from build123d import *

# Parameters (mm, degrees)
CROQUIS1_W               = 100
CROQUIS1_H               = 15
SALIENTE_EXTRUIR1_DEPTH  = 50
CROQUIS17_R              = 30
CORTAR_EXTRUIR1_DEPTH    = 15
BARRER1_PROFILE_R        = 35
CORTAR_BARRER2_PROFILE_R = 30
REDONDEO1_R              = 15
TALADRO1_D               = 15
TALADRO1_DEPTH           = 15
CROQUIS26_W              = 100
CROQUIS26_H              = 100
SALIENTE_EXTRUIR3_DEPTH  = 15
REDONDEO2_R              = 15
CROQUIS29_R              = 30
CORTAR_EXTRUIR2_DEPTH    = 15
TALADRO2_D               = 15
TALADRO2_DEPTH           = 15
TALADRO2_ON_FACE_2_D     = 15
TALADRO2_ON_FACE_2_DEPTH = 15


with BuildPart() as part:
    # Croquis1 → Saliente-Extruir1 (new, symmetric)
    with BuildSketch(Plane.XY):
        with Locations((0, 7.5)):
            Rectangle(CROQUIS1_W, CROQUIS1_H)
    extrude(amount=SALIENTE_EXTRUIR1_DEPTH, both=True)

    # Croquis17 → Cortar-Extruir1 (cut)
    with BuildSketch(Plane(origin=(0, 15, 0), x_dir=(1, 0, 0), z_dir=(0, 1, 0))):
        with Locations(Location((0, 0, 0), (0, 0, 180))):
            Circle(CROQUIS17_R)
    extrude(amount=-CORTAR_EXTRUIR1_DEPTH, mode=Mode.SUBTRACT)

    # Barrer1: sweep along a path in Croquis2
    with BuildLine(Plane.XY) as barrer1_path:
        Line((0, 0), (0, 61.152236891))
        ThreePointArc((0, 61.152236891), (9.895660774, 110.901083099), (38.076118446, 153.076118446))
        Line((38.076118446, 153.076118446), (70.710678119, 185.710678119))
    # Barrer1 profile (on start of the path) → Barrer1 (sweep)
    with BuildSketch(Plane(origin=(0, 0, 0), x_dir=(1, 0, 0), z_dir=(0, 1, 0))):
        Circle(BARRER1_PROFILE_R)
    sweep(path=barrer1_path.line)

    # Cortar-Barrer2: sweep along a path in Croquis2<5>
    with BuildLine(Plane.XY) as cortar_barrer2_path:
        Line((0, 0), (0, 61.152236891))
        ThreePointArc((0, 61.152236891), (9.895660774, 110.901083099), (38.076118446, 153.076118446))
        Line((38.076118446, 153.076118446), (70.710678119, 185.710678119))
    # Cortar-Barrer2 profile (on start of the path) → Cortar-Barrer2 (sweep, cut)
    with BuildSketch(Plane(origin=(0, 0, 0), x_dir=(1, 0, 0), z_dir=(0, 1, 0))):
        Circle(CORTAR_BARRER2_PROFILE_R)
    sweep(path=cortar_barrer2_path.line, mode=Mode.SUBTRACT)

    # Redondeo1
    redondeo1_edges = [part.edges().sort_by_distance(p)[0] for p in [
        (50, 7.5, 50),
        (-50, 7.5, 50),
        (50, 7.5, -50),
        (-50, 7.5, -50),
    ]]
    fillet(redondeo1_edges, radius=REDONDEO1_R)

    # Taladro1
    with Locations(Plane(origin=(-35, 15, -35), x_dir=(1, 0, 0), z_dir=(0, 1, 0))):
        with Locations((0, 0), (0, -70), (70, 0), (70, -70)):
            Hole(TALADRO1_D / 2, depth=TALADRO1_DEPTH)

    # Croquis26 → Saliente-Extruir3 (add)
    with BuildSketch(Plane(origin=(128.210678119, 128.210678119, 0), x_dir=(0, 0, -1), z_dir=(0.7071067811865478, 0.7071067811865472, 0))):
        with Locations((0, 81.317279836)):
            Rectangle(CROQUIS26_W, CROQUIS26_H)
    extrude(amount=SALIENTE_EXTRUIR3_DEPTH)

    # Redondeo2
    redondeo2_edges = [part.edges().sort_by_distance(p)[0] for p in [
        (40.658639918, 226.369318037, 50),
        (111.369318037, 155.658639918, 50),
        (111.369318037, 155.658639918, -50),
        (40.658639918, 226.369318037, -50),
    ]]
    fillet(redondeo2_edges, radius=REDONDEO2_R)

    # Croquis29 → Cortar-Extruir2 (cut)
    with BuildSketch(Plane(origin=(138.817279836, 138.817279836, 0), x_dir=(0, 0, -1), z_dir=(0.7071067811865479, 0.7071067811865472, 0))):
        with Locations(Location((0, 81.317279836, 0), (0, 0, 90))):
            Circle(CROQUIS29_R)
    extrude(amount=-CORTAR_EXTRUIR2_DEPTH, mode=Mode.SUBTRACT)

    # Taladro2
    with Locations(Plane(origin=(56.568542495, 221.066017178, 35), x_dir=(-0.707106781187, 0.707106781187, 0), z_dir=(0.707106781187, 0.707106781187, 0))):
        with Locations((0, 0)):
            Hole(TALADRO2_D / 2, depth=TALADRO2_DEPTH)

    # Taladro2 on face 2
    with Locations(Plane(origin=(106.066017178, 171.568542495, 35), x_dir=(0.707106781187, -0.707106781187, 0), z_dir=(0.707106781187, 0.707106781187, 0))):
        with Locations((0, 0), (0, 70), (-70, 70)):
            Hole(TALADRO2_ON_FACE_2_D / 2, depth=TALADRO2_ON_FACE_2_DEPTH)


solid = part.part
Build history of the part. All positions in model axes, mm. A direction names the side the tool comes from. Give positions to 0.01 mm unless a question says otherwise; leave off trailing zeros. Loops run counter-clockwise (first coordinate to the right, second up) from the corner with the lowest first, then second, coordinate; pieces in that order, holes last. Notation, with made-up numbers: (62, 34) -> (80, 34) arc R27 ccw to (80, 55) -> close; hole circle Ø11 at (-28.5, 29.5). An arc over 180 degrees is marked (long way). Answer in a Markdown table with one row per item.
Item 1: Slice it at B-B on y = 45. Write the cut outline in (x, z), plus the area to 3 significant figures.
Findings below:
| item | result |
|---|---|
| outline | circle Ø70 at (0, 0); hole circle Ø60 at (0, 0) |
| area | 1,020 mm² |
Item 2: Probe line 1 along Z through (x, y) = (-35, 4); line 2 along Y through (x, z) = (44, -2.5). List the from-to ranges inside material, lowest first. Write a range as [from, to].
Findings below:
| item | result |
|---|---|
| line 1 | z = [-50, -42.5], [-27.5, 27.5], [42.5, 50] |
| line 2 | y = [0, 15], [101.72, 112.39], [201.28, 208.37], [212.42, 229.71] |
Item 3: Mould opens along Z. For faces 5 (the cylindrical face through (36.63, 7.4, -27.68)), 6 (the cylindrical face through (108.42, 158.76, -45.49)), 7 (the cylindrical face through (108.254, 158.922, 45.723)) say: pulls with the +Z half, pulls with the -Z half, needs draft (parallel to the pull), parting line crosses it, or undercut.
Findings below:
| item | result |
|---|---|
| face 5 | undercut |
| face 6 | pulls with the -Z half |
| face 7 | pulls with the +Z half |
Item 4: Flat gauge pins, fed straight in: P1, Ø1.5, axis at y = 64.5, z = 24, coming from the -X side; P2, Ø1, axis at y = 141.5, z = -25.5, coming from the +X side; P3, Ø13.5, axis at x = -35, z = -35, coming from the +Y side; P4, Ø10, axis at x = -5, y = 118.5, coming from the +Z side. Where does each tip first touch, or does it go through?
Findings below:
| item | result |
|---|---|
| P1 | stops at x = -26.13 |
| P2 | stops at x = 61.3 |
| P3 | passes through |
| P4 | stops at z = 33 |
Item 5: Slice it at A-A on z = -8.5. Write the cut outline in (x, y), plus the area to 3 significant figures.
Findings below:
| item | result |
|---|---|
| outline | (-50, 0) -> (-28.77, 0) -> (-28.77, 61.15) arc R158.77 cw to (17.73, 173.42) -> (60.97, 216.66) -> (45.96, 231.67) -> (35.36, 221.07) -> (46.7, 209.72) -> (14.07, 177.08) arc R163.95 ccw to (-33.95, 61.15) -> (-33.95, 15) -> (-50, 15) -> close; (28.77, 0) -> (50, 0) -> (50, 15) -> (33.95, 15) -> (33.95, 61.15) arc R96.05 cw to (62.08, 129.07) -> (94.72, 161.7) -> (106.07, 150.36) -> (116.67, 160.96) -> (101.66, 175.97) -> (58.42, 132.73) arc R101.23 ccw to (28.77, 61.15) -> close |
| area | 3,290 mm² |
Item 6: Tool access for faces 1 (the flat face through (-50, 7, 0)), 2 (the flat face through (50, 7, 0)), 3 (the flat face through (46.645, 209.776, 11.811)), 4 (the cylindrical face through (45.49, 7.6, 45.72)): list every direction of +Z, -Z, +X, -X, +Y, -Y with a clear straight run to the whole face (end or side of a thin tool).
Findings below:
| item | result |
|---|---|
| face 1 | +Z, -Z, -X, +Y, -Y |
| face 2 | +Z, -Z, +X, -Y |
| face 3 | none |
| face 4 | +Z, +X, -Y |
